The model under review builds one solid part; all positions refer to its coordinate system, in mm. Face numbers are marked on the shaded views. A direction names the side the tool comes from. Round coordinates to 2 decimals unless told otherwise and drop trailing zeros. Write each loop counter-clockwise with the first axis right and the second up, starting at its lowest first coordinate (ties: lowest second). Pieces come first, ordered by that corner, then holes. Notation, with made-up numbers: (16.25, 53.5) - (68.25, 53.5) arc R23 ccw to (68.25, 70.5) - close; hole circle Ø9 at (-23.5, 71.5). An arc over 180 degrees is marked (long way). Return JSON: item names as keys, results as strings.
from build123d import *

# Parameters (mm, degrees)
F0_R     = 2.7
F1_DEPTH = 9
F3_DEPTH = 2.6
F4_W     = 9.5
F4_H     = 9
F5_DEPTH = 3.8
F6_R     = 1.6
F7_DEPTH = 9


with BuildPart() as f1:
    # F0 (on Top) → F1 (new body)
    with BuildSketch(Plane.XY):
        with BuildLine():
            ThreePointArc((0, 4.75), (3.358757, 3.358757), (4.75, 0))
            Line((4.75, 0), (4.75, 4.75))
            Line((4.75, 4.75), (0, 4.75))
        make_face()
        with BuildLine():
            ThreePointArc((-4.75, 0), (-3.358757, 3.358757), (0, 4.75))
            Line((0, 4.75), (-4.75, 4.75))
            Line((-4.75, 4.75), (-4.75, 0))
        make_face()
        with BuildLine():
            ThreePointArc((-4.75, 0), (0, -4.75), (4.75, 0))
            ThreePointArc((4.75, 0), (3.358757, 3.358757), (0, 4.75))
            ThreePointArc((0, 4.75), (-3.358757, 3.358757), (-4.75, 0))
        make_face()
        Circle(F0_R, mode=Mode.SUBTRACT)
    extrude(amount=F1_DEPTH)

    # F2 (on face) → F3 (join)
    with BuildSketch(Plane(origin=(0, 4.75, 0), x_dir=(-1, 0, 0), z_dir=(0, 1, 0))):
        Polygon((-4.75, 7.4), (-1.674316, 7.4), (1.674316, 7.4), (3.348632, 4.5), (1.674316, 1.6), (-1.674316, 1.6), (-4.75, 1.6), (-4.75, 0), (4.75, 0), (4.75, 9), (-4.75, 9), align=None)
    extrude(amount=F3_DEPTH)

    # F4 (on face) → F5 (join)
    with BuildSketch(Plane(origin=(0, 7.35, 0), x_dir=(-1, 0, 0), z_dir=(0, 1, 0))):
        with Locations((0, 4.5)):
            Rectangle(F4_W, F4_H)
    extrude(amount=F5_DEPTH)

    # F6 (on face) → F7 (cut)
    with BuildSketch(Plane(origin=(0, 11.15, 0), x_dir=(-1, 0, 0), z_dir=(0, 1, 0))):
        with Locations((0, 4.5)):
            Circle(F6_R)
    extrude(amount=-F7_DEPTH, mode=Mode.SUBTRACT)


solid = f1.part
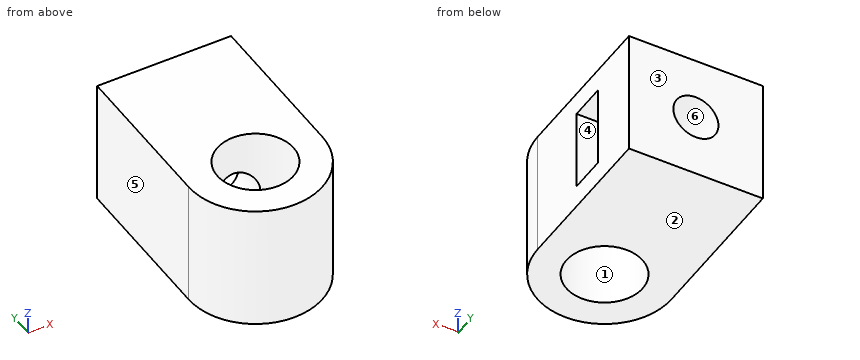
(1) Add section B-B (z = 3.75). Write out the cut boundary in (x, y).
Filled in:
{"outline": "(-4.75, 0) arc R4.75 ccw to (4.75, 0) - (4.75, 4.75) - (1.41, 4.75) - (1.41, 2.3) arc R2.7 cw (long way) to (-1.41, 2.3) - (-1.41, 4.75) - (-2.92, 4.75) - (-2.92, 7.35) - (-1.41, 7.35) - (-1.41, 11.15) - (-4.75, 11.15) - close; (1.41, 7.35) - (4.75, 7.35) - (4.75, 11.15) - (1.41, 11.15) - close"}
(2) Mouldability with a two-part tool opening along Y and no side actions: class the marked faces 1, 2, 3 and 4 as released by +Y, released by -Y, zero draft, split by the parting line, or undercut.
Filled in:
{"face 1": "undercut", "face 2": "zero draft", "face 3": "released by +Y", "face 4": "undercut"}
(3) Clearance check with flat-ended pins moving along their axes: pin 1 Ø1.9 at (x, z) = (0, 4.5) entering from +Y; pin 2 Ø2 at (x, z) = (-3, 4.5) entering from -Y. State where each tip first meets the part, or that it passes through.
Filled in:
{"pin 1": "stops at y = -2.53", "pin 2": "stops at y = -4.31"}
(4) Add section D-D (x = -2.25). Write out the cut boundary in (y, z), plus the area to 3 significant figures.
Filled in:
{"outline": "(-4.18, 0) - (-1.49, 0) - (-1.49, 9) - (-4.18, 9) - close; (1.49, 0) - (11.15, 0) - (11.15, 9) - (1.49, 9) - close; hole (4.75, 2.6) - (7.35, 2.6) - (7.35, 6.4) - (4.75, 6.4) - close", "area": "101 mm2"}
(5) Add section C-C (y = 4). Write out the cut boundary in (x, z), plus the area to 3 significant figures.
Filled in:
{"outline": "(-4.75, 0) - (4.75, 0) - (4.75, 9) - (-4.75, 9) - close; hole circle Ø3.2 at (0, 4.5)", "area": "77.5 mm2"}
(6) Wall thickness on line 1 (Z direction, x = 0, y = 3.1); line 2 (Y direction, x = -1.5, z = 3) (3 decimals); line 3 (X direction, y = 3.1, z = 4.5): over which ranges is each line inside the solid? List them lowest first.
Filled in:
{"line 1": "z = 0 to 2.9, 6.1 to 9", "line 2": "y = -4.507 to -2.245, 2.245 to 4.75, 7.35 to 11.15", "line 3": "x = -4.75 to -1.6, 1.6 to 4.75"}
(7) For the marked faces 5 and 6, list the 3-axis set-ups (+Z, -Z, +X, -X, +Y, -Y) from which the entire face can be reached by the end or side of a thin tool; tool diameter is ignored.
Filled in:
{"face 5": "+Z, -Z, -X, +Y, -Y", "face 6": "+Y"}
(8) Add section A-A (x = 0). Write out the cut boundary in (y, z).
Filled in:
{"outline": "(-4.75, 0) - (-2.7, 0) - (-2.7, 9) - (-4.75, 9) - close; (2.7, 0) - (11.15, 0) - (11.15, 2.9) - (7.35, 2.9) - (7.35, 1.6) - (4.75, 1.6) - (4.75, 2.9) - (2.7, 2.9) - close; (2.7, 6.1) - (4.75, 6.1) - (4.75, 7.4) - (7.35, 7.4) - (7.35, 6.1) - (11.15, 6.1) - (11.15, 9) - (2.7, 9) - close"}
